Verification items for the finished model (mm, model axes). A direction names the side the tool comes from. Coordinates: 2 decimals unless noted, no trailing zeros. Write each loop counter-clockwise with the first axis right and the second up, starting at its lowest first coordinate (ties: lowest second). Pieces come first, ordered by that corner, then holes. Notation, with made-up numbers: (53.5, -12) - (73.5, -12) arc R17 ccw to (73.5, 16) - close; hole circle Ø6 at (-3.75, -27). An arc over 180 degrees is marked (long way). Answer as CSV lines item,"result". Start each with the question number.
```python
from build123d import *

# Parameters (mm, degrees)
BOSS_EXTRUDE1_DEPTH      = 12.5
BOSS_EXTRUDE1_DEPTH_BACK = 12.5


with BuildPart() as part:
    # Sketch3 → Boss-Extrude1 (new, two sides: drawn at the far end of the back side and taken through both)
    with BuildSketch(Plane.XY.offset(-BOSS_EXTRUDE1_DEPTH_BACK)):
        with BuildLine():
            Line((41.209392703, -4.902647552), (25.123270681, -152.873223024))
            ThreePointArc((25.123270681, -152.873223024), (26.308155139, -162.131131278), (31.56629724, -169.842470855))
            Line((31.56629724, -169.842470855), (94.847375791, -227.248960885))
            ThreePointArc((94.847375791, -227.248960885), (115.02027127, -235.027885849), (135.182633585, -227.221700382))
            Line((135.182633585, -227.221700382), (215.312641305, -154.332733182))
            ThreePointArc((215.312641305, -154.332733182), (247.701260572, -157.830965895), (239.450301839, -189.3457556))
            Line((239.450301839, -189.3457556), (185.765566437, -217.299410382))
            ThreePointArc((185.765566437, -217.299410382), (175.163893091, -232.519848612), (181.632970164, -249.90398677))
            Line((181.632970164, -249.90398677), (232.737634385, -295.843508488))
            ThreePointArc((232.737634385, -295.843508488), (244.347239065, -332.377604686), (216.900021711, -359.139020295))
            Line((216.900021711, -359.139020295), (54.051747266, -395.534867829))
            ThreePointArc((54.051747266, -395.534867829), (31.510113512, -394.280366061), (12.960804924, -381.410938028))
            Line((12.960804924, -381.410938028), (-71.598619136, -278.699186983))
            ThreePointArc((-71.598619136, -278.699186983), (-76.490286444, -265.680265539), (-72.389705453, -252.390948019))
            Line((-72.389705453, -252.390948019), (-33.571850395, -196.429497877))
            ThreePointArc((-33.571850395, -196.429497877), (-30.74094047, -190.403305276), (-30.045757005, -183.781691559))
            Line((-30.045757005, -183.781691559), (-41.395449867, -2.943931093))
            ThreePointArc((-41.395449867, -2.943931093), (0.983766669, 41.488338158), (41.209392703, -4.902647552))
        make_face()
        with BuildLine():
            Line((39.758565065, -4.322218299), (23.650555587, -152.494128769))
            ThreePointArc((23.650555587, -152.494128769), (24.861691641, -162.563897665), (30.554318883, -170.958008173))
            Line((30.554318883, -170.958008173), (93.835397434, -228.364498202))
            ThreePointArc((93.835397434, -228.364498202), (115.24071321, -236.533134868), (136.518688321, -228.038316235))
            Line((136.518688321, -228.038316235), (216.545640027, -155.243092274))
            ThreePointArc((216.545640027, -155.243092274), (246.399107149, -158.594576746), (239.234433563, -187.768698837))
            Line((239.234433563, -187.768698837), (185.549698161, -215.722353619))
            ThreePointArc((185.549698161, -215.722353619), (173.674724909, -232.298612729), (180.981535847, -251.335363232))
            Line((180.981535847, -251.335363232), (232.031793649, -297.225977381))
            ThreePointArc((232.031793649, -297.225977381), (242.840884818, -332.189452533), (216.571433386, -357.668796481))
            Line((216.571433386, -357.668796481), (53.72315894, -394.064644015))
            ThreePointArc((53.72315894, -394.064644015), (31.999811145, -392.855682033), (14.123862745, -380.453428312))
            Line((14.123862745, -380.453428312), (-70.435561315, -277.741677267))
            ThreePointArc((-70.435561315, -277.741677267), (-74.976572908, -265.856709803), (-71.428149605, -253.638611342))
            Line((-71.428149605, -253.638611342), (-32.610294547, -197.6771612))
            ThreePointArc((-32.610294547, -197.6771612), (-29.330340619, -190.951417289), (-28.554164527, -183.508885489))
            Line((-28.554164527, -183.508885489), (-39.91427806, -2.505089621))
            ThreePointArc((-39.91427806, -2.505089621), (0.911894069, 39.982415088), (39.758565065, -4.322218299))
        make_face(mode=Mode.SUBTRACT)
    extrude(amount=BOSS_EXTRUDE1_DEPTH + BOSS_EXTRUDE1_DEPTH_BACK)


solid = part.part
```
1. Draft check along X on faces 5 (the face through (-27.56, -329.82, -0.18)), 6 (the face through (244.48, -331.83, -0.18)), 7 (the face through (-53.25, -224.8, -0.18)). Enter one of: pulls with the +X half, pulls with the -X half, needs draft (parallel to the pull), parting line crosses it, or undercut.
2. Cross-section at D-D (y = -55.5). Record the cut outline in (x, z), and give its area (3 significant figures).
3. Scan lines: line 1 along Y through (x, z) = (206, 6.75); line 2 along X through (y, z) = (-182, 7.75); line 3 along X through (y, z) = (-230, 7.5). Record each from-to range of solid material in increasing order. Write a range as from..to.
4. Cross-section at B-B (y = -164.5). Record the cut outline in (x, z).
5. Access from +Z, -Z, +X, -X, +Y, -Y to the whole of each face (thin tool, end or side, straight path). Record for faces 1 (the face through (-35.64, -94.63, -0.18)), 2 (the face through (-34.155, -94.274, -0.175)), 3 (the face through (206.828, -272.552, -0.175)), 4 (the face through (31.813, -394.383, -0.175)).
6. Depth check by flat-ended pin: P1, Ø1.5, axis at x = 205, z = 3, coming from the -Y side; P2, Ø24, axis at x = 230, y = -170.03, coming from the +Z side; P3, Ø12, axis at y = -350, z = -4.5, coming from the +X side; P4, Ø4, axis at y = -103, z = 2, coming from the -X side. Enter the tip coordinate at first touch or a pass-through.
7. Cross-section at C-C (x = 209). Record the cut outline in (y, z), and give its area (3 significant figures).
8. Cross-section at A-A (x = 117). Record the cut outline in (y, z), and give its area (3 significant figures).
Completed:
1,face 5,"undercut"
1,face 6,"pulls with the +X half"
1,face 7,"pulls with the -X half"
2,outline,"(-38.1, -12.5) - (-36.59, -12.5) - (-36.59, 12.5) - (-38.1, 12.5) - close; (34.19, -12.5) - (35.71, -12.5) - (35.71, 12.5) - (34.19, 12.5) - close"
2,area,"75.6 mm2"
3,line 1,"y = -361.58..-360.03, -273.83..-271.81, -206.76..-205.07, -164.84..-162.8"
3,line 2,"x = -30.16..-28.65, 42.73..44.97, 184.9..187.13, 246.02..247.86"
3,line 3,"x = -56.86..-55.03, 95.79..98.38, 131.62..134.21, 174.1..175.65"
4,outline,"(-31.26, -12.5) - (-29.75, -12.5) - (-29.75, 12.5) - (-31.26, 12.5) - close; (25.7, -12.5) - (27.39, -12.5) - (27.39, 12.5) - (25.7, 12.5) - close; (204.14, -12.5) - (206.37, -12.5) - (206.37, 12.5) - (204.14, 12.5) - close; (249.21, -12.5) - (250.78, -12.5) - (250.78, 12.5) - (249.21, 12.5) - close"
5,face 1,"+Z, -Z, -X"
5,face 2,"+Z, -Z"
5,face 3,"+Z, -Z, +X"
5,face 4,"+Z, -Z, -Y"
6,P1,"stops at y = -361.97"
6,P2,"passes through"
6,P3,"stops at x = 239.15"
6,P4,"stops at x = -35.24"
7,outline,"(-360.9, -12.5) - (-359.36, -12.5) - (-359.36, 12.5) - (-360.9, 12.5) - close; (-276.52, -12.5) - (-274.51, -12.5) - (-274.51, 12.5) - (-276.52, 12.5) - close; (-205.2, -12.5) - (-203.51, -12.5) - (-203.51, 12.5) - (-205.2, 12.5) - close; (-162.11, -12.5) - (-160.07, -12.5) - (-160.07, 12.5) - (-162.11, 12.5) - close"
7,area,"182 mm2"
8,outline,"(-381.47, -12.5) - (-379.92, -12.5) - (-379.92, 12.5) - (-381.47, 12.5) - close; (-236.47, -12.5) - (-234.96, -12.5) - (-234.96, 12.5) - (-236.47, 12.5) - close"
8,area,"76.3 mm2"
